Autodesk Inventor part; units mm, degrees
ref_plane "XYPlane" through (14.8, 16.3, 3.6) normal (0, 1, 0) x (1, 0, 0)
ref_plane "YZPlane" through (13.3, 11.0574, 3.6) normal (-1, 0, 0) x (0, 0, 1)
ref_plane "LeftLine" through (8.3, 11.0574, 3.6) normal (1, 0, 0) x (0, 0, -1)
sketch "Sketch1" plane through (0, 0, 0) normal (0, 0, 1) x (1, 0, 0)
  line L0 (0, 0) -> (26.6, 0)
  line L1 (26.6, 0) -> (26.6, 26.6)
  line L2 (26.6, 26.6) -> (0, 26.6)
  line L3 (0, 26.6) -> (0, 0)
  dimension "d0" = 26.6
  dimension "d1" = 26.6
extrude "Extrusion1" add sketch "Sketch1" along normal blind 3.6
chamfer "Chamfer1" distance 2 angle 45 4 edges at (13.3, 26.6, 0) (0, 13.3, 0) (26.6, 13.3, 0) (13.3, 0, 0)
sketch "Sketch2" plane through (0, 0, 0) normal (0, 0, -1) x (-1, 0, 0)
  line L0 (0, 26.6) -> (0, 0) construction
  line L1 (0, 20.5614) -> (-6, 20.5614) construction
  line L2 (-26.6, 26.6) -> (0, 26.6) construction
  line L3 (-7.1317, 26.6) -> (-7.1317, 21.9) construction
  line L4 (-7.1317, 26.6) -> (-2.4317, 26.6) construction
  line L5 (-6, 21.9) -> (-8.5, 21.9) construction
  line L6 (-8.5, 21.9) -> (-8.5, 14.8) construction
  line L7 (-8.5, 14.8) -> (-6, 14.8) construction
  line L8 (-6, 14.8) -> (-6, 21.9) construction
  line L9 (-13.3, 26.6) -> (-13.3, 0) construction
  line L10 (0, 0) -> (-26.6, 0) construction
  line L11 (-20.6, 21.9) -> (-18.1, 21.9) construction
  line L12 (-18.1, 21.9) -> (-18.1, 14.8) construction
  line L13 (-18.1, 14.8) -> (-20.6, 14.8) construction
  line L14 (-20.6, 14.8) -> (-20.6, 21.9) construction
  line L15 (-13.3, 0) -> (-13.3, 4) construction
  line L16 (-13.3, 4) -> (-10.8, 4) construction
  line L17 (-10.8, 4) -> (-15.8, 4) construction
  line L18 (-15.8, 4) -> (-15.8, 9) construction
  line L19 (-15.8, 9) -> (-10.8, 9) construction
  line L20 (-10.8, 9) -> (-10.8, 4) construction
  line L21 (-15.8, 4) -> (-15.8, 7) construction
  line L22 (-10.8, 4) -> (-10.8, 7) construction
  arc A0 (-10.8, 7) -> (-15.8, 7) centre (-13.3, 6.4375) ccw construction
  line L23 (-20.6, 21.9) -> (-18.1, 21.9)
  line L24 (-18.1, 21.9) -> (-18.1, 14.8)
  line L25 (-18.1, 14.8) -> (-20.6, 14.8)
  line L26 (-20.6, 14.8) -> (-20.6, 21.9)
  line L27 (-8.5, 21.9) -> (-6, 21.9)
  line L28 (-6, 21.9) -> (-6, 14.8)
  line L29 (-6, 14.8) -> (-8.5, 14.8)
  line L30 (-8.5, 14.8) -> (-8.5, 21.9)
  line L31 (-15.8, 4) -> (-10.8, 4)
  line L32 (-10.8, 7) -> (-10.8, 4)
  line L33 (-15.8, 4) -> (-15.8, 7)
  arc A1 (-10.8, 7) -> (-15.8, 7) centre (-13.3, 6.4375) ccw
  dimension "d7" = 6
  dimension "d9" = 4.7
  dimension "d11" = 2.5
  dimension "d12" = 7.1
  dimension "d13" = 4
  dimension "d14" = 2.5
  dimension "d15" = 5
  dimension "d16" = 5
  dimension "d17" = 3
extrude "Extrusion2" cut sketch "Sketch2" against normal blind 3.6
sketch "Sketch3" plane through (0, 0, 3.6) normal (0, 0, 1) x (1, 0, 0)
  line L0 (15.8, 4) -> (10.8, 4) construction
  line L1 (10.8, 4) -> (10.8, 7) construction
  arc A0 (15.8, 7) -> (10.8, 7) centre (13.3, 6.4375) ccw construction
  line L2 (15.8, 7) -> (15.8, 4) construction
  line L3 (6, 14.8) -> (6, 21.9) construction
  line L4 (6, 21.9) -> (8.5, 21.9) construction
  line L5 (8.5, 21.9) -> (8.5, 14.8) construction
  line L6 (8.5, 14.8) -> (6, 14.8) construction
  line L7 (18.1, 14.8) -> (18.1, 21.9) construction
  line L8 (18.1, 21.9) -> (20.6, 21.9) construction
  line L9 (20.6, 21.9) -> (20.6, 14.8) construction
  line L10 (20.6, 14.8) -> (18.1, 14.8) construction
  line L11 (26.6, 0) -> (26.6, 26.6) construction
  line L12 (26.6, 26.6) -> (0, 26.6) construction
  line L13 (0, 26.6) -> (0, 0) construction
  line L14 (0, 0) -> (26.6, 0) construction
  line L15 (13.3, 26.6) -> (13.3, 0) construction
  line L16 (4.8, 2.55) -> (21.8, 2.55) construction
  line L17 (21.8, 2.55) -> (21.8, 24.05) construction
  line L18 (21.8, 24.05) -> (4.8, 24.05) construction
  line L19 (4.8, 24.05) -> (4.8, 2.55) construction
  line L20 (4.8, 2.55) -> (21.8, 24.05) construction
  line L21 (21.8, 2.55) -> (4.8, 24.05) construction
  line L22 (21.8, 2.55) -> (17.4, 2.55) construction
  line L23 (17.4, 2.55) -> (17.4, 8.55) construction
  line L24 (17.4, 8.55) -> (21.8, 8.55) construction
  line L25 (21.8, 8.55) -> (21.8, 2.55) construction
  line L26 (4.8, 2.55) -> (9.2, 2.55) construction
  line L27 (9.2, 2.55) -> (9.2, 8.55) construction
  line L28 (9.2, 8.55) -> (4.8, 8.55) construction
  line L29 (4.8, 8.55) -> (4.8, 2.55) construction
  line L30 (11.8, 37.0426) -> (14.8, 37.0426) construction
  line L31 (14.8, 37.0426) -> (14.8, 11.0574) construction
  line L32 (14.8, 11.0574) -> (11.8, 11.0574) construction
  line L33 (11.8, 11.0574) -> (11.8, 37.0426) construction
  line L34 (11.8, 37.0426) -> (14.8, 11.0574) construction
  line L35 (14.8, 37.0426) -> (11.8, 11.0574) construction
  line L36 (4.8, 24.05) -> (11.8, 24.05)
  line L37 (11.8, 11.0574) -> (11.8, 24.05)
  line L38 (11.8, 11.0574) -> (14.8, 11.0574)
  line L39 (14.8, 11.0574) -> (14.8, 24.05)
  line L40 (14.8, 24.05) -> (21.8, 24.05)
  line L41 (21.8, 24.05) -> (21.8, 8.55)
  line L42 (21.8, 8.55) -> (17.4, 8.55)
  line L43 (17.4, 8.55) -> (17.4, 2.55)
  line L44 (17.4, 2.55) -> (9.2, 2.55)
  line L45 (9.2, 2.55) -> (9.2, 8.55)
  line L46 (9.2, 8.55) -> (4.8, 8.55)
  line L47 (4.8, 8.55) -> (4.8, 24.05)
  point P0 (13.3, 13.3)
  point P1 (13.3, 24.05)
  dimension "d20" = 17
  dimension "d21" = 21.5
  dimension "d22" = 4.4
  dimension "d23" = 6
  dimension "d24" = 4.4
  dimension "d25" = 6
  dimension "d26" = 3
extrude "Extrusion3" add sketch "Sketch3" along normal blind 20
chamfer "Chamfer2" distance 1 angle 45 4 edges at (4.8, 24.05, 13.6) (21.8, 24.05, 13.6) (17.4, 2.55, 13.6) (9.2, 2.55, 13.6)
fillet "Fillet1" radius 0.5 13 edges at (8.8, 24.05, 23.6) (4.8, 15.8, 23.6) (11.8, 17.5537, 23.6) (14.8, 17.5537, 23.6) (17.8, 24.05, 23.6) (21.8, 15.8, 23.6) (19.6, 8.55, 23.6) (17.4, 6.05, 23.6) (9.2, 6.05, 23.6) (7, 8.55, 23.6) (13.3, 2.55, 23.6) (21.3, 23.55, 23.6) (5.3, 23.55, 23.6)
sketch "Sketch4" plane through (14.8, 16.3, 3.6) normal (0, 1, 0) x (1, 0, 0)
  line L0 (-10, 0) -> (-10, -19.5) construction
  line L1 (11.8, 0) -> (-14.8, 0) construction
  line L2 (-8.7929, -20) -> (-3.5, -20) construction
  arc A0 (-3.5, -20) -> (-3, -19.5) centre (-3.5, -19.5) ccw construction
  line L3 (-3, -19.5) -> (-9, -19.5) construction
  ellipse E0 centre (-8.7929, -19.5) end of major axis (-8.7929, -20) minor radius 0.2071 (-9, -19.5) -> (-8.7929, -20) ccw construction
  line L4 (-9.5, -20) -> (-8.7929, -20) construction
  ellipse E1 centre (-8.7929, -19.5) end of major axis (-8.7929, -20) minor radius 0.2071 (-9, -19.5) -> (-8.7929, -20) ccw construction
  line L5 (-9, -19.5) -> (-10, -19.5) construction
  arc A1 (-10, -19.5) -> (-9.5, -20) centre (-9.5, -19.5) ccw construction
  line L6 (-7.8516, -20) -> (-7.8516, -17.5) construction
  line L7 (-7.8516, -17.5) -> (-16.9269, -17.5) construction
  line L8 (-10, -3.8087) -> (-15, -3.8087) construction
  line L9 (-14.8, 0) -> (-14.8, -3) construction
  line L10 (-10, 0) -> (-11.6, 0) construction
  line L11 (-11.6, 0) -> (-14.8, -3) construction
  line L12 (-10, -17.5) -> (-12, -17.5) construction
  line L13 (-12, -17.5) -> (-14.8, -3) construction
  arc A2 (-12.3892, -15.4843) -> (-10, -17.5) centre (-10.1078, -15.204) ccw construction
  arc A3 (-12.3892, -15.4843) -> (-10, -17.5) centre (-10.1078, -15.204) ccw
  line L14 (-12.3892, -15.4843) -> (-14.8, -3)
  line L15 (-14.8, -3) -> (-11.6, 0)
  line L16 (-11.6, 0) -> (-10, 0)
  line L17 (-10, 0) -> (-10, -17.5)
  point P0 (-14.8, 3.6)
  dimension "d33" = 2.5
  dimension "d34" = 5
  dimension "d35" = 3
  dimension "d36" = 1.6
  dimension "d37" = 2
extrude "Extrusion4" add sketch "Sketch4" along normal blind 7.3 and the other way blind 3.65
mirror "Mirror1" about plane through (13.3, 11.0574, 3.6) normal (-1, 0, 0) of "Extrusion4"
ref_plane "LeftLine" through (8.3, 11.0574, 3.6) normal (1, 0, 0) x (0, 0, -1)
sketch "Sketch5" plane through (8.3, 11.0574, 3.6) normal (1, 0, 0) x (0, 0, -1)
  line L0 (-20, -2.0074) -> (-20, 11.7855) construction
  line L1 (-19.5, 12.9926) -> (0, 12.9926) construction
  line L2 (-20, 11.7855) -> (-20, 12.4926) construction
  line L3 (0, -2.5074) -> (-19.5, -2.5074) construction
  line L4 (-20, 12.9926) -> (-13.6632, 12.9926) construction
  line L5 (-13.6632, 12.9926) -> (-13.6632, -2.5074) construction
  line L6 (-13.6632, -2.5074) -> (-20, -2.5074) construction
  line L7 (-20, -2.5074) -> (-20, 12.9926) construction
  line L8 (-20, 12.9926) -> (-20, 11.9926) construction
  line L9 (-20, -2.5074) -> (-20, 2.4926) construction
  line L10 (-20, 2.4926) -> (-23, 2.4926) construction
  line L11 (-23, 2.4926) -> (-23, 11.9926) construction
  line L12 (-23, 11.9926) -> (-20, 11.9926) construction
  line L13 (-20, 11.9926) -> (-20, 2.4926) construction
  line L14 (-23, 11.9926) -> (-20, 11.9926)
  line L15 (-20, 11.9926) -> (-20, 2.4926)
  line L16 (-20, 2.4926) -> (-23, 2.4926)
  line L17 (-23, 2.4926) -> (-23, 11.9926)
  point P0 (3.6, -11.0574)
  dimension "d42" = 1
  dimension "d43" = 5
  dimension "d44" = 3
extrude "Extrusion5" add sketch "Sketch5" along normal mid plane 0.35
chamfer "Chamfer3" distance 1 angle 45 2 edges at (8.3, 23.05, 26.6) (8.3, 13.55, 26.6)
mirror "Mirror2" about plane through (13.3, 11.0574, 3.6) normal (-1, 0, 0) of "Extrusion5", "Chamfer3"
chamfer "Chamfer4" distance 0.5 angle 45 12 edges at (19.35, 21.9, 0) (18.1, 18.35, 0) (20.6, 18.35, 0) (19.35, 14.8, 0) (7.25, 14.8, 0) (6, 18.35, 0) (7.25, 21.9, 0) (8.5, 18.35, 0) (13.3, 9, 0) (15.8, 5.5, 0) (10.8, 5.5, 0) (13.3, 4, 0)
properties part number "Plug"
The listing builds one solid part. Answer for the finished solid, in the listing's coordinates (mm). A direction names the side the tool comes from. Round coordinates to 2 decimals unless told otherwise and drop trailing zeros. Order: outer loops, then holes, each group sorted by start corner. A loop starts at its lowest first (then second) coordinate and runs counter-clockwise, first axis right, second up. Notation, with made-up numbers: M 1,7.25 L 33,7.25 A18 ccw 33,24.25 Z; hole C 75,-15 d6. An arc over 180 degrees is marked long. Answer in a Markdown table with one row per item. Add a question column.
1) The part is cut by section A-A on z = 22.5. Determine the outline of the cut face in (x, y), plus the area to 3 significant figures.
2) The part is cut by section D-D on y = 10.25. Determine the outline of the cut face in (x, z).
3) Consider line 1 along X through (y, z) = (23, 21.25); line 2 along Z through (x, y) = (9.5, 18.75); line 3 along X through (y, z) = (10.75, 6.25). Determine where each line is inside the solid, lowest interval first. Write a range as from..to.
4) The part is cut by section C-C on x = 7.5. Determine the outline of the cut face in (y, z).
5) The part is cut by section B-B on y = 5. Determine the outline of the cut face in (x, z).
6) Determine the mould class of faces 5 (the face through (14.8, 17, 13)), 6 (the face through (16.91, 3.06, 13.74)), 7 (the face through (13, 7, 3.6)) for opening direction Y: pulls with the +Y half, pulls with the -Y half, needs draft (parallel to the pull), parting line crosses it, or undercut.
7) Which of the six approach directions +Z, -Z, +X, -X, +Y, -Y give full straight-line access (tool end or side, diameter ignored) to faces 1 (the face through (8.475, 18, 25)), 2 (the face through (10.8, 6, 2)), 3 (the face through (8.125, 18, 25)), 4 (the face through (13, 2.55, 13))?
8) Flat-ended cylindrical pins translate along their axes: pin 1 Ø4 at (x, z) = (24, 12.5) entering from -Y; pin 2 Ø7 at (y, z) = (17, 9.5) entering from -X; pin 3 Ø1.5 at (y, z) = (19, 25) entering from -X (3 decimals). Find the tip coordinate at first contact, or state that the pin passes through.
Findings below:
| question | item | result |
|---|---|---|
| 1 | outline | M 4.8,8.55 L 9.2,8.55 L 9.2,3.55 L 10.2,2.55 L 16.4,2.55 L 17.4,3.55 L 17.4,8.55 L 21.8,8.55 L 21.8,23.05 L 20.8,24.05 L 14.8,24.05 L 14.8,11.06 L 11.8,11.06 L 11.8,24.05 L 5.8,24.05 L 4.8,23.05 Z |
| 1 | area | 272 mm² |
| 2 | outline | M 0,2 L 2,0 L 24.6,0 L 26.6,2 L 26.6,3.6 L 21.8,3.6 L 21.8,23.1 A0.5 ccw 21.3,23.6 L 5.3,23.6 A0.5 ccw 4.8,23.1 L 4.8,3.6 L 0,3.6 Z |
| 3 | line 1 | x = 4.8..11.8, 14.8..21.8 |
| 3 | line 2 | z = 0..23.6 |
| 3 | line 3 | x = 4.8..21.8 |
| 4 | outline | M 0,2 L 2,0 L 14.3,0 L 14.8,0.5 L 14.8,3.6 L 21.9,3.6 L 21.9,0.5 L 22.4,0 L 24.6,0 L 26.6,2 L 26.6,3.6 L 24.05,3.6 L 24.05,23.1 A0.5 ccw 23.55,23.6 L 9.05,23.6 A0.5 ccw 8.55,23.1 L 8.55,3.6 L 0,3.6 Z |
| 5 | outline | M 0,2 L 2,0 L 10.3,0 L 10.8,0.5 L 10.8,3.6 L 15.8,3.6 L 15.8,0.5 L 16.3,0 L 24.6,0 L 26.6,2 L 26.6,3.6 L 17.4,3.6 L 17.4,23.1 A0.5 ccw 16.9,23.6 L 9.7,23.6 A0.5 ccw 9.2,23.1 L 9.2,3.6 L 0,3.6 Z |
| 6 | face 5 | needs draft |
| 6 | face 6 | pulls with the -Y half |
| 6 | face 7 | undercut |
| 7 | face 1 | +Z, +Y, -Y |
| 7 | face 2 | -Z |
| 7 | face 3 | +Z, -X, +Y, -Y |
| 7 | face 4 | +Z, +X, -X, -Y |
| 8 | pin 1 | stops at y = 12.65 |
| 8 | pin 2 | stops at x = 0 |
| 8 | pin 3 | stops at x = 8.125 |
